Source: CAD feature listing. Evaluate the final solid. Frame: model axes, mm. Face numbers are marked on the shaded views. A direction names the side the tool comes from. Round coordinates to 2 decimals unless told otherwise and drop trailing zeros. Loops run counter-clockwise (first coordinate to the right, second up) from the corner with the lowest first, then second, coordinate; pieces in that order, holes last. Notation, with made-up numbers: M 24.5,-21.75 L 53.5,-21.75 A22 ccw 53.5,14.25 Z; hole C 89,-26.5 d3. An arc over 180 degrees is marked long. Answer as a JSON object with one key per item and string values.
from build123d import *

# Parameters (mm, degrees)
BARRA_START         = -32.5
SK_BARRA_W          = 41
SK_BARRA_H          = 9
BARRA_DEPTH         = 5
EXTREMOS_START      = -32.5
SK_EXTREMOS_R       = 4.5
EXTREMOS_DEPTH      = 5
PERNO_696_START     = -39.5
SK_PERNO_696_R      = 2.975
PERNO_696_DEPTH     = 7
PASANTES_M2_5_START = -32.5
SK_PASANTES_M2_5_R  = 1.45
PASANTES_M2_5_DEPTH = 5
CAJAS_M2_5_START    = -32.5
SK_CAJAS_M2_5_R     = 2.5
CAJAS_M2_5_DEPTH    = 2.7


with BuildPart() as part:
    # Sk_Barra → Barra (new body)
    with BuildSketch(Plane(origin=(0, 0, 0), x_dir=(1, 0, 0), z_dir=(0, 1, 0)).offset(BARRA_START)):
        with Locations((0, -490)):
            Rectangle(SK_BARRA_W, SK_BARRA_H)
    extrude(amount=BARRA_DEPTH)

    # Sk_Extremos → Extremos (add)
    with BuildSketch(Plane(origin=(0, 0, 0), x_dir=(1, 0, 0), z_dir=(0, 1, 0)).offset(EXTREMOS_START)):
        with Locations((-20.5, -490)):
            Circle(SK_EXTREMOS_R)
        with Locations((20.5, -490)):
            Circle(SK_EXTREMOS_R)
    extrude(amount=EXTREMOS_DEPTH)

    # Sk_Perno_696 → Perno_696 (add)
    with BuildSketch(Plane(origin=(0, 0, 0), x_dir=(1, 0, 0), z_dir=(0, 1, 0)).offset(PERNO_696_START)):
        with Locations(Location((0, -490, 0), (0, 0, 270))):
            Circle(SK_PERNO_696_R)
    extrude(amount=PERNO_696_DEPTH)

    # Sk_Pasantes_M2-5 → Pasantes_M2-5 (cut)
    with BuildSketch(Plane(origin=(0, 0, 0), x_dir=(1, 0, 0), z_dir=(0, 1, 0)).offset(PASANTES_M2_5_START)):
        with Locations(Location((-20.5, -490, 0), (0, 0, 270))):
            Circle(SK_PASANTES_M2_5_R)
        with Locations(Location((20.5, -490, 0), (0, 0, 270))):
            Circle(SK_PASANTES_M2_5_R)
    extrude(amount=PASANTES_M2_5_DEPTH, mode=Mode.SUBTRACT)

    # Sk_Cajas_M2-5 → Cajas_M2-5 (cut)
    with BuildSketch(Plane(origin=(0, 0, 0), x_dir=(1, 0, 0), z_dir=(0, 1, 0)).offset(CAJAS_M2_5_START)):
        with Locations(Location((-20.5, -490, 0), (0, 0, 270))):
            Circle(SK_CAJAS_M2_5_R)
        with Locations(Location((20.5, -490, 0), (0, 0, 270))):
            Circle(SK_CAJAS_M2_5_R)
    extrude(amount=CAJAS_M2_5_DEPTH, mode=Mode.SUBTRACT)


solid = part.part
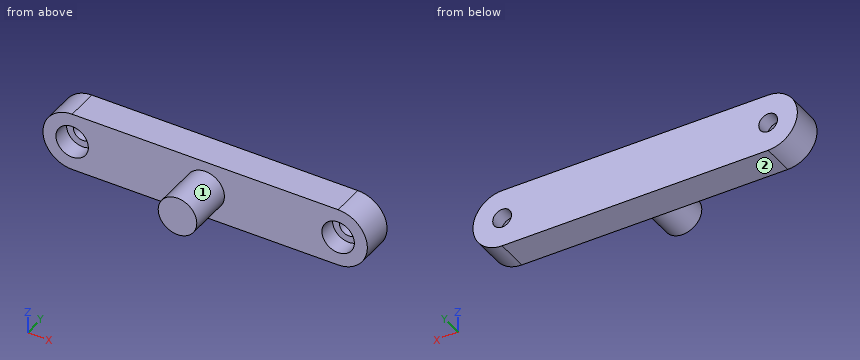
Item 1: Section A-A on z = 490. Return the cut outline in (x, y) (3 decimals).
Answer sheet:
{"outline": "M -25,-32.5 L -23,-32.5 L -23,-29.8 L -21.95,-29.8 L -21.95,-27.5 L -25,-27.5 Z; M -19.05,-29.8 L -18,-29.8 L -18,-32.5 L -2.975,-32.5 L -2.975,-39.5 L 2.975,-39.5 L 2.975,-32.5 L 18,-32.5 L 18,-29.8 L 19.05,-29.8 L 19.05,-27.5 L -19.05,-27.5 Z; M 21.95,-29.8 L 23,-29.8 L 23,-32.5 L 25,-32.5 L 25,-27.5 L 21.95,-27.5 Z"}
Item 2: Section B-B on x = 0. Return the cut outline in (y, z) (3 decimals).
Answer sheet:
{"outline": "M -39.5,487.025 L -32.5,487.025 L -32.5,485.5 L -27.5,485.5 L -27.5,494.5 L -32.5,494.5 L -32.5,492.975 L -39.5,492.975 Z"}
Item 3: Line query: probe 1 along X at (y, z) = (-28.65, 490); probe 2 along X at (y, z) = (-31.7, 490); probe 3 along Z at (x, y) = (20.5, -28.5). Output: solid intervals per line, ascending. Write a range as from..to.
Answer sheet:
{"probe 1": "x = -25..-21.95, -19.05..19.05, 21.95..25", "probe 2": "x = -25..-23, -18..18, 23..25", "probe 3": "z = 485.5..488.55, 491.45..494.5"}
Item 4: Section C-C on y = -36. Return the cut outline in (x, z) (3 decimals), then the cut area to 3 significant figures.
Answer sheet:
{"outline": "C 0,490 d5.95", "area": "27.8 mm²"}
Item 5: Contact query for flat-ended pins moving along their axis: pin 1 Ø2.5 at (x, z) = (-20.5, 491) entering from -Y; pin 2 Ø1 at (y, z) = (-30, 486.5) entering from +X; pin 3 Ø5 at (y, z) = (-36.5, 492.5) entering from +X (3 decimals). Output: stop coordinate, or through.
Answer sheet:
{"pin 1": "stops at y = -29.8", "pin 2": "stops at x = 23.85", "pin 3": "stops at x = 2.975"}
Item 6: Section D-D on z = 492. Return the cut outline in (x, y), then the cut area to 3 significant figures.
Answer sheet:
{"outline": "M -24.53,-32.5 L -22,-32.5 L -22,-29.8 L -19,-29.8 L -19,-32.5 L -2.2,-32.5 L -2.2,-39.5 L 2.2,-39.5 L 2.2,-32.5 L 19,-32.5 L 19,-29.8 L 22,-29.8 L 22,-32.5 L 24.53,-32.5 L 24.53,-27.5 L -24.53,-27.5 Z", "area": "260 mm²"}
Item 7: Access query for the marked faces 1 and 2. Directions: +Z, -Z, +X, -X, +Y, -Y. A direction counts if a zero-diameter tool reaches every point of the face in a straight line with its end or side. Return the directions, or none.
Answer sheet:
{"face 1": "-Y", "face 2": "-Z, +X, -X, +Y, -Y"}
